from build123d import *

# Parameters (mm, degrees)
BLANKSKE_W          = 95
BLANKSKE_H          = 11
BLANK_DEPTH         = 5.5
TOOTHCUTSIM_DEPTH   = 96.792745028
TEETHCUTS_COUNT     = 27
TEETHCUTS_PITCH     = 3.14159265
SKETCH_1_W          = 10
SKETCH_1_H          = 5
CUT_EXTRUDE_1_DEPTH = 96.792745028


with BuildPart() as part:
    # BlankSke → Blank (new body)
    with BuildSketch(Plane.XY):
        with Locations((47.5, 5.5)):
            Rectangle(BLANKSKE_W, BLANKSKE_H)
    extrude(amount=-BLANK_DEPTH)

    # TooCutSkeSim → ToothCutSim (cut, through all)
    with BuildSketch(Plane.XY):
        Polygon((0.44443537, 8.75), (-0.44443537, 8.75), (-1.272613241, 11.0254), (1.272613241, 11.0254), align=None)
    toothcutsim = extrude(amount=-TOOTHCUTSIM_DEPTH, mode=Mode.SUBTRACT)

    # TeethCuts: ToothCutSim ×27
    with Locations(*[(i * TEETHCUTS_PITCH, 0, 0) for i in range(1, TEETHCUTS_COUNT)]):
        add(toothcutsim, mode=Mode.SUBTRACT)

    # ｽｹｯﾁ1 → ｶｯﾄ - 押し出し1 (cut, through all)
    with BuildSketch(Plane(origin=(0, 0, -5.5), x_dir=(-1, 0, 0), z_dir=(0, 0, -1))):
        with Locations((-97.5, 2.5)):
            Rectangle(SKETCH_1_W, SKETCH_1_H)
        with Locations((2.5, 2.5)):
            Rectangle(SKETCH_1_W, SKETCH_1_H)
        with Locations((-17.5, 2.5)):
            Rectangle(SKETCH_1_W, SKETCH_1_H)
        with Locations((-37.5, 2.5)):
            Rectangle(SKETCH_1_W, SKETCH_1_H)
        with Locations((-57.5, 2.5)):
            Rectangle(SKETCH_1_W, SKETCH_1_H)
        with Locations((-77.5, 2.5)):
            Rectangle(SKETCH_1_W, SKETCH_1_H)
    extrude(amount=-CUT_EXTRUDE_1_DEPTH, mode=Mode.SUBTRACT)


solid = part.part
Work out the finished part from the listing and answer in its coordinate system (mm). A direction names the side the tool comes from. Round coordinates to 2 decimals unless told otherwise and drop trailing zeros. Write each loop counter-clockwise with the first axis right and the second up, starting at its lowest first coordinate (ties: lowest second). Pieces come first, ordered by that corner, then holes. Notation, with made-up numbers: (-21, 12.25) -> (30, 12.25) arc R17 cw to (30, 41.25) -> close; hole circle Ø8 at (35, 82.25). An arc over 180 degrees is marked (long way). Answer as CSV lines item,"result". Start each with the question number.
(1) Each of these flat-tipped pins is pushed along its axis until it touches: pin 1 (1.5 mm diameter, centred on y = 3.5, z = -2, fed in from +X); pin 2 (2 mm diameter, centred on y = 2.5, z = -3, fed in from -X). Where does it stop, or does it pass through?
(2) Find the intervals of material crossed by probe 1 along X at (y, z) = (3.5, -4.9); probe 2 along Y at (x, z) = (9, -1.9); probe 3 along Y at (x, z) = (39.5, -3.55), in increasing order.
(3) A tool of negligible diameter and unlimited length cuts with its end or side. For faces 4 (the flat face through (94, 5, -3)), 5 (the flat face through (44.84, 9.89, -2.71)), 6 (the flat face through (42.5, 2, -3)), from which of +Z, -Z, +X, -X, +Y, -Y can it reach the whole face along a straight path? Write none if from no direction.
(4) The part is cut by section A-A, the plane y = 4. Give the vertices of the cut face in (x, z), then the cut area to 3 significant figures.
(5) The mould has two halves that part along X. Classify faces 1 (the flat face through (47, 6, -5.5)), 2 (the flat face through (30.568, 9.859, -2.712)), 3 (the flat face through (38, 5, -3)): +X half, -X half, draft (parallel to the pull), parting line (faces both ways), or undercut.
Output values:
1,pin 1,"stops at x = 92.5"
1,pin 2,"stops at x = 2.5"
2,probe 1,"x = 2.5 to 12.5, 22.5 to 32.5, 42.5 to 52.5, 62.5 to 72.5, 82.5 to 92.5"
2,probe 2,"y = 0 to 8.75"
2,probe 3,"y = 5 to 11"
3,face 4,"+Z, -Z, +X, -Y"
3,face 5,"+Z, -Z, +Y"
3,face 6,"+Z, -Z, -Y"
4,outline,"(2.5, -5.5) -> (12.5, -5.5) -> (12.5, 0) -> (2.5, 0) -> close; (22.5, -5.5) -> (32.5, -5.5) -> (32.5, 0) -> (22.5, 0) -> close; (42.5, -5.5) -> (52.5, -5.5) -> (52.5, 0) -> (42.5, 0) -> close; (62.5, -5.5) -> (72.5, -5.5) -> (72.5, 0) -> (62.5, 0) -> close; (82.5, -5.5) -> (92.5, -5.5) -> (92.5, 0) -> (82.5, 0) -> close"
4,area,"275 mm²"
5,face 1,"draft"
5,face 2,"undercut"
5,face 3,"undercut"
